```python
from build123d import *

# Parameters (mm, degrees)
BOSS_EXTRUDE1_DEPTH      = 110
BOSS_EXTRUDE1_DEPTH_BACK = 110
SKETCH1_W                = 15
SKETCH1_H                = 15
SKETCH2_R                = 4
BOSS_EXTRUDE2_DEPTH      = 35
BOSS_EXTRUDE3_START      = 35
SKETCH3_R                = 4
BOSS_EXTRUDE3_DEPTH      = 35
BOSS_EXTRUDE4_DEPTH      = 7.5
BOSS_EXTRUDE4_DEPTH_BACK = 7.5
SKETCH5_R                = 6
CUT_EXTRUDE1_DEPTH       = 157.888495435
SKETCH6_R                = 5
CUT_EXTRUDE5_DEPTH       = 20
SKETCH7_R                = 12.5
CUT_EXTRUDE2_DEPTH       = 5
FILLET2_R                = 30
CHAMFER1_SIZE            = 2


with BuildPart() as part:
    # Sketch1 → Boss-Extrude1 (new, two sides: drawn at the far end of the back side and taken through both)
    with BuildSketch(Plane.XY.offset(-BOSS_EXTRUDE1_DEPTH_BACK)):
        Rectangle(SKETCH1_W, SKETCH1_H)
    extrude(amount=BOSS_EXTRUDE1_DEPTH + BOSS_EXTRUDE1_DEPTH_BACK)

    # Sketch2 → Boss-Extrude2 (add)
    with BuildSketch(Plane.XY.offset(110)):
        Circle(SKETCH2_R)
    extrude(amount=BOSS_EXTRUDE2_DEPTH)

    # Sketch3 → Boss-Extrude3 (add)
    with BuildSketch(Plane(origin=(0, 0, -110), x_dir=(-1, 0, 0), z_dir=(0, 0, -1)).offset(BOSS_EXTRUDE3_START)):
        with Locations(Location((0, 0, 0), (0, 0, 180))):
            Circle(SKETCH3_R)
    extrude(amount=-BOSS_EXTRUDE3_DEPTH)

    # Sketch4 → Boss-Extrude4 (add, two sides: drawn at the far end of the back side and taken through both)
    with BuildSketch(Plane(origin=(0, 0, 0), x_dir=(0, 0, -1), z_dir=(1, 0, 0)).offset(-BOSS_EXTRUDE4_DEPTH_BACK)):
        Polygon((-30, 7.5), (-7.5, 58), (7.5, 58), (30, 7.5), align=None)
    extrude(amount=BOSS_EXTRUDE4_DEPTH + BOSS_EXTRUDE4_DEPTH_BACK)

    # Sketch5 → Cut-Extrude1 (cut, through all)
    with BuildSketch(Plane(origin=(7.5, 0, 0), x_dir=(0, 0, -1), z_dir=(1, 0, 0))):
        with Locations((0, 18)):
            Circle(SKETCH5_R)
    extrude(amount=-CUT_EXTRUDE1_DEPTH, mode=Mode.SUBTRACT)

    # Sketch6 → Cut-Extrude5 (cut)
    with BuildSketch(Plane(origin=(0, 58, 0), x_dir=(1, 0, 0), z_dir=(0, 1, 0))):
        with Locations(Location((0, 0, 0), (0, 0, 270))):
            Circle(SKETCH6_R)
    extrude(amount=-CUT_EXTRUDE5_DEPTH, mode=Mode.SUBTRACT)

    # Sketch7 → Cut-Extrude2 (cut)
    with BuildSketch(Plane(origin=(7.5, 0, 0), x_dir=(0, 0, -1), z_dir=(1, 0, 0))):
        with Locations((0, 18)):
            Circle(SKETCH7_R)
    cut_extrude2 = extrude(amount=-CUT_EXTRUDE2_DEPTH, mode=Mode.SUBTRACT)

    # Mirror1: Cut-Extrude2 across plane
    add(cut_extrude2.mirror(Plane(origin=(0, 0, 0), x_dir=(0, 0, 1), z_dir=(1, 0, 0))), mode=Mode.SUBTRACT)

    # Fillet2
    fillet2_edges = [part.edges().sort_by_distance(p)[0] for p in [
        (0, 7.5, -30),
        (0, 7.5, 30),
    ]]
    fillet(fillet2_edges, radius=FILLET2_R)

    # Chamfer1
    chamfer1_edges = [part.edges().sort_by_distance(p)[0] for p in [
        (-7.5, 41.645338647, 14.786730306),
        (-7.5, 58, 0),
        (7.5, 58, 0),
        (7.5, 41.645338647, 14.786730306),
        (7.5, 18, 12.5),
        (-7.5, 18, 12.5),
        (7.5, 41.645338647, -14.786730306),
        (-7.5, 41.645338647, -14.786730306),
        (-7.5, 7.5, 79.738303565),
        (-7.5, 7.5, -79.738303565),
        (7.5, 7.5, 79.738303565),
        (7.5, 7.5, -79.738303565),
        (7.5, 12.33772982, -33.140752104),
        (-7.5, 12.33772982, -33.140752104),
        (7.5, -7.5, 0),
        (7.5, 12.33772982, 33.140752104),
        (-7.5, 12.33772982, 33.140752104),
        (-7.5, -7.5, 0),
    ]]
    chamfer(chamfer1_edges, length=CHAMFER1_SIZE)


solid = part.part
```
The listing builds one solid part. Answer for the finished solid, in the listing's coordinates (mm). A direction names the side the tool comes from. Give positions to 0.01 mm unless a question says otherwise; leave off trailing zeros. Write each loop counter-clockwise with the first axis right and the second up, starting at its lowest first coordinate (ties: lowest second). Pieces come first, ordered by that corner, then holes. Notation, with made-up numbers: (88.25, 36.25) - (113.25, 36.25) arc R11 cw to (113.25, 55.25) - close; hole circle Ø3 at (87.25, 38). An arc over 180 degrees is marked (long way). Use one line per item in the form item = value. Start each with the question number.
1) Find section B-B on y = 0. Determine the outline of the cut face in (x, z).
2) A tool of negligible diameter and unlimited length cuts with its end or side. For faces 5 (the face through (4.02, 6.91, -5.77)), 6 (the face through (-2.5, 12.6, 3)), 7 (the face through (0, 7.5, 79)), from which of +Z, -Z, +X, -X, +Y, -Y can it reach the whole face along a straight path? Write none if from no direction.
3) Find section D-D on y = 48. Determine the outline of the cut face in (x, z).
4) Find section C-C on x = 0. Determine the outline of the cut face in (y, z), plus the area to 3 significant figures.
5) Flat-ended cylindrical pins translate along their axes: pin 1 Ø15 at (y, z) = (18, 0) entering from +X; pin 2 Ø3.5 at (x, z) = (0, 84.5) entering from +Y; pin 3 Ø2 at (x, y) = (2.5, 15) entering from -Z. Find the tip coordinate at first contact, or state that the pin passes through.
6) Find section A-A on z = 0. Determine the outline of the cut face in (x, y), plus the area to 4 significant figures.
7) The mould has two halves that part along Z. Classify faces 1 (the face through (2.5, 12.6, 3)), 2 (the face through (0, 38, 0)), 3 (the face through (5.625, 12.366, -32.869)), 4 (the face through (0, 7.5, -80)): pulls with the +Z half, pulls with the -Z half, needs draft (parallel to the pull), parting line crosses it, or undercut.
8) Consider line 1 along Y through (x, z) = (4.5, 0); line 2 along Y through (x, z) = (0.05, 0); line 3 along Y through (x, z) = (-1.5, -76). Determine where each line is inside the solid, lowest interval first. Write a range as from..to.
Geometry results:
q1.outline = (-7.5, -110) - (-4, -110) - (-4, -145) - (4, -145) - (4, -110) - (7.5, -110) - (7.5, 110) - (4, 110) - (4, 145) - (-4, 145) - (-4, 110) - (-7.5, 110) - close
q2.face_5 = +X
q2.face_6 = -X
q2.face_7 = +Z, +X, -X, +Y
q3.outline = (-7.5, -9.77) - (-5.5, -11.96) - (5.5, -11.96) - (7.5, -9.77) - (7.5, 9.77) - (5.5, 11.96) - (-5.5, 11.96) - (-7.5, 9.77) - close; hole circle Ø10 at (0, 0)
q4.outline = (-7.5, -110) - (-4, -110) - (-4, -145) - (4, -145) - (4, -110) - (7.5, -110) - (7.5, -49.48) arc R30 cw to (25.29, -22.07) - (58, -7.5) - (58, -5) - (38, -5) - (38, 5) - (58, 5) - (58, 7.5) - (25.29, 22.07) arc R30 cw to (7.5, 49.48) - (7.5, 110) - (4, 110) - (4, 145) - (-4, 145) - (-4, 110) - (-7.5, 110) - close; hole circle Ø12 at (18, 0)
q4.area = 5,570 mm2
q5.pin_1 = 2.5
q5.pin_2 = 7.5
q5.pin_3 = -30.83
q6.outline = (-7.5, -5.5) - (-5.5, -7.5) - (5.5, -7.5) - (7.5, -5.5) - (7.5, 3.5) - (5.5, 5.5) - (2.5, 5.5) - (2.5, 12) - (-2.5, 12) - (-2.5, 5.5) - (-5.5, 5.5) - (-7.5, 3.5) - close; (-7.5, 32.5) - (-5.5, 30.5) - (-2.5, 30.5) - (-2.5, 24) - (2.5, 24) - (2.5, 30.5) - (5.5, 30.5) - (7.5, 32.5) - (7.5, 56) - (5.5, 58) - (5, 58) - (5, 38) - (-5, 38) - (-5, 58) - (-5.5, 58) - (-7.5, 56) - close
q6.area = 456.5 mm2
q7.face_1 = undercut
q7.face_2 = undercut
q7.face_3 = pulls with the -Z half
q7.face_4 = needs draft
q8.line_1 = -7.5..5.5, 30.5..38
q8.line_2 = -7.5..12, 24..38
q8.line_3 = -7.5..7.5
